Can you work these out from the model? Positions are in its coordinate system, mm. Face numbers are marked on the shaded views. Give positions to 0.01 mm unless a question says otherwise; leave off trailing zeros. Write each loop counter-clockwise with the first axis right and the second up, starting at its lowest first coordinate (ties: lowest second). Pieces come first, ordered by that corner, then holes.
```python
from build123d import *

# Parameters (mm, degrees)
F0_W     = 12
F0_H     = 12
F1_DEPTH = 4
F2_D     = 4
F2_DEPTH = 2
F2_TIP   = 1.2017212381
F3_R     = 3


with BuildPart() as f1:
    # F0 (on Top) → F1 (new body)
    with BuildSketch(Plane.XY):
        Rectangle(F0_W, F0_H)
    extrude(amount=F1_DEPTH)

    # F2
    with Locations(Plane(origin=(0, 0, 0), x_dir=(1, 0, 0), z_dir=(0, 0, -1))):
        with Locations((0, 0)):
            Hole(F2_D / 2, depth=F2_DEPTH)
            with Locations((0, 0, -(F2_DEPTH + F2_TIP / 2))):  # 118° drill point
                Cone(0, F2_D / 2, F2_TIP, mode=Mode.SUBTRACT)

    # F3
    f3_edges = [f1.edges().sort_by_distance(p)[0] for p in [
        (6, 6, 2),
        (-6, 6, 2),
        (-6, -6, 2),
        (6, -6, 2),
    ]]
    fillet(f3_edges, radius=F3_R)


solid = f1.part
```
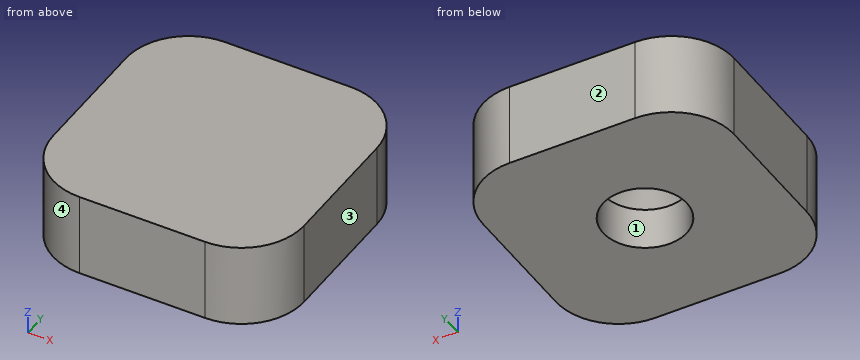
1) Suppose I cut it at C-C on y = 4.5. Write out the boundary of the cut face in (x, z), plus the area to 3 significant figures.
Values follow:
outline: (-5.6, 0) - (5.6, 0) - (5.6, 4) - (-5.6, 4) - close
area: 44.8 mm2
2) Please list where these lines run through material, in increasing order: L1, parallel to Y at x = 0, z = 1.45; L2, parallel to X at y = -0.5, z = 2.25; L3, parallel to X at y = 0.5, z = 2.2.
Values follow:
L1: y = -6 to -2, 2 to 6
L2: x = -6 to -1.5, 1.5 to 6
L3: x = -6 to -1.59, 1.59 to 6
3) Suppose I cut it at D-D on x = 4. Write out the boundary of the cut face in (y, z).
Values follow:
outline: (-5.83, 0) - (5.83, 0) - (5.83, 4) - (-5.83, 4) - close
4) If we mould it in two halves opening along Y, with no side actions, what happens to the marked faces 1, 2, 3 and 4? For each: +Y half, -Y half, draft (parallel to the pull), parting line (faces both ways), or undercut.
Values follow:
face 1: undercut
face 2: +Y half
face 3: draft
face 4: -Y half
5) Suppose I cut it at A-A on z = 1.6. Write out the boundary of the cut face in (x, y).
Values follow:
outline: (-6, -3) arc R3 ccw to (-3, -6) - (3, -6) arc R3 ccw to (6, -3) - (6, 3) arc R3 ccw to (3, 6) - (-3, 6) arc R3 ccw to (-6, 3) - close; hole circle Ø4 at (0, 0)
6) For pin 1 Ø1.5 at (y, z) = (-4.5, 3) entering from -X, with a flat end and sliding along its axis, tell me the tip position at first contact or that it passes through.
Values follow:
pin 1: stops at x = -5.9
7) Suppose I cut it at B-B on z = 3.65. Write out the boundary of the cut face in (x, y), plus the area to 3 significant figures.
Values follow:
outline: (-6, -3) arc R3 ccw to (-3, -6) - (3, -6) arc R3 ccw to (6, -3) - (6, 3) arc R3 ccw to (3, 6) - (-3, 6) arc R3 ccw to (-6, 3) - close
area: 136 mm2
